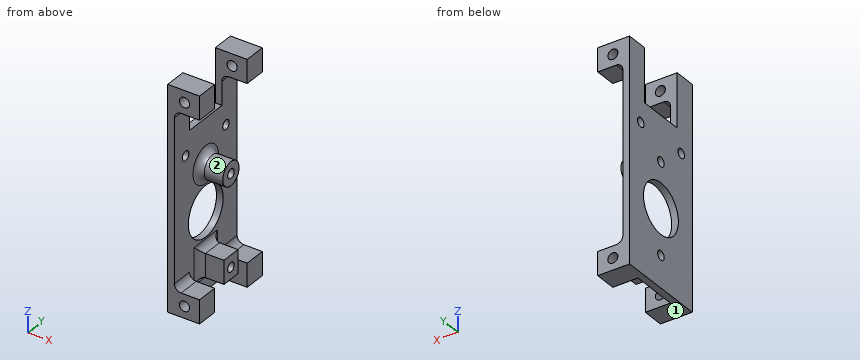
```python
from build123d import *

# Parameters (mm, degrees)
SKETCH1_W           = 66
SKETCH1_H           = 27
BOSS_EXTRUDE1_DEPTH = 2
SKETCH2_R           = 7.5
CUT_EXTRUDE1_DEPTH  = 2
BOSS_EXTRUDE2_DEPTH = 7.5
SKETCH4_R           = 1.5
CUT_EXTRUDE2_DEPTH  = 31
SKETCH5_R           = 1.4
CUT_EXTRUDE3_DEPTH  = 31
SKETCH6_W           = 7
SKETCH6_H           = 27
BOSS_EXTRUDE3_DEPTH = 7.5
SKETCH7_R           = 1.5
CUT_EXTRUDE4_DEPTH  = 33.5
SKETCH8_W           = 16
SKETCH8_H           = 14
CUT_EXTRUDE5_DEPTH  = 15.75
SKETCH9_R           = 1.4
CUT_EXTRUDE6_DEPTH  = 31.5
SKETCH10_R          = 3.5
BOSS_EXTRUDE4_DEPTH = 7.5
SKETCH11_R          = 1.4
CUT_EXTRUDE7_DEPTH  = 9.5
CUT_EXTRUDE8_DEPTH  = 7.5
FILLET1_R           = 2


with BuildPart() as part:
    # Sketch1 → Boss-Extrude1 (new body)
    with BuildSketch(Plane(origin=(0, 0, 0), x_dir=(0, 0, -1), z_dir=(1, 0, 0))):
        Rectangle(SKETCH1_W, SKETCH1_H)
    extrude(amount=BOSS_EXTRUDE1_DEPTH)

    # Sketch2 → Cut-Extrude1 (cut)
    with BuildSketch(Plane(origin=(2, 0, 0), x_dir=(0, 0, -1), z_dir=(1, 0, 0))):
        with Locations((10, 0)):
            Circle(SKETCH2_R)
    extrude(amount=-CUT_EXTRUDE1_DEPTH, mode=Mode.SUBTRACT)

    # Sketch3 → Boss-Extrude2 (add)
    with BuildSketch(Plane(origin=(2, 0, 0), x_dir=(0, 0, -1), z_dir=(1, 0, 0))):
        Polygon((33, 13.5), (26, 13.5), (26, 3), (20, 3), (20, -3), (26, -3), (26, -13.5), (33, -13.5), align=None)
    extrude(amount=BOSS_EXTRUDE2_DEPTH)

    # Sketch4 → Cut-Extrude2 (cut)
    with BuildSketch(Plane(origin=(0, 13.5, 0), x_dir=(1, 0, 0), z_dir=(0, 1, 0))):
        with Locations(Location((5, 29.5, 0), (0, 0, 270))):
            Circle(SKETCH4_R)
    extrude(amount=-CUT_EXTRUDE2_DEPTH, mode=Mode.SUBTRACT)

    # Sketch5 → Cut-Extrude3 (cut)
    with BuildSketch(Plane(origin=(9.5, 0, 0), x_dir=(0, 0, -1), z_dir=(1, 0, 0))):
        with Locations((23.54, 0)):
            Circle(SKETCH5_R)
    extrude(amount=-CUT_EXTRUDE3_DEPTH, mode=Mode.SUBTRACT)

    # Sketch6 → Boss-Extrude3 (add)
    with BuildSketch(Plane(origin=(2, 0, 0), x_dir=(0, 0, -1), z_dir=(1, 0, 0))):
        with Locations((-29.5, 0)):
            Rectangle(SKETCH6_W, SKETCH6_H)
    extrude(amount=BOSS_EXTRUDE3_DEPTH)

    # Sketch7 → Cut-Extrude4 (cut)
    with BuildSketch(Plane(origin=(0, 13.5, 0), x_dir=(1, 0, 0), z_dir=(0, 1, 0))):
        with Locations(Location((5, -29.5, 0), (0, 0, 270))):
            Circle(SKETCH7_R)
    extrude(amount=-CUT_EXTRUDE4_DEPTH, mode=Mode.SUBTRACT)

    # Sketch8 → Cut-Extrude5 (cut, symmetric)
    with BuildSketch(Plane(origin=(2, 0, 0), x_dir=(0, 0, -1), z_dir=(1, 0, 0))):
        with Locations((-25, 0)):
            Rectangle(SKETCH8_W, SKETCH8_H)
    extrude(amount=CUT_EXTRUDE5_DEPTH, both=True, mode=Mode.SUBTRACT)

    # Sketch9 → Cut-Extrude6 (cut)
    with BuildSketch(Plane(origin=(2, 0, 0), x_dir=(0, 0, -1), z_dir=(1, 0, 0))):
        with Locations((-10.5, -8.7)):
            Circle(SKETCH9_R)
    cut_extrude6 = extrude(amount=-CUT_EXTRUDE6_DEPTH, mode=Mode.SUBTRACT)

    # Mirror1: Cut-Extrude6 across plane
    add(cut_extrude6.mirror(Plane.ZX), mode=Mode.SUBTRACT)

    # Sketch10 → Boss-Extrude4 (add)
    with BuildSketch(Plane(origin=(2, 0, 0), x_dir=(0, 0, -1), z_dir=(1, 0, 0))):
        with Locations(Location((-3.54, 0, 0), (0, 0, 180))):
            Circle(SKETCH10_R)
    extrude(amount=BOSS_EXTRUDE4_DEPTH)

    # Sketch11 → Cut-Extrude7 (cut)
    with BuildSketch(Plane(origin=(9.5, 0, 0), x_dir=(0, 0, -1), z_dir=(1, 0, 0))):
        with Locations((-3.54, 0)):
            Circle(SKETCH11_R)
    extrude(amount=-CUT_EXTRUDE7_DEPTH, mode=Mode.SUBTRACT)

    # Sketch12 → Cut-Extrude8 (cut)
    with BuildSketch(Plane(origin=(9.5, 0, 0), x_dir=(0, 0, -1), z_dir=(1, 0, 0))):
        Polygon((26, -7), (33, -7), (33, -3), (33, 3), (33, 7), (26, 7), (26, 3), (27, 3), (27, -3), (26, -3), align=None)
    extrude(amount=-CUT_EXTRUDE8_DEPTH, mode=Mode.SUBTRACT)

    # Fillet1
    fillet1_edges = [part.edges().sort_by_distance(p)[0] for p in [
        (2, 0, 0.04),
        (2, -10.25, 26),
        (2, -10.25, -26),
        (2, 0, -20),
        (2, -3, -23.5),
        (2, 3, -23.5),
        (2, 10.25, -26),
        (2, 10.25, 26),
        (2, 0, -27),
    ]]
    fillet(fillet1_edges, radius=FILLET1_R)


solid = part.part
```
CAD build for the part. Positions are in the model's coordinates, mm. Face numbers are marked on the shaded views. A direction names the side the tool comes from. Round coordinates to 2 decimals unless told otherwise and drop trailing zeros. Order: outer loops, then holes, each group sorted by start corner. A loop starts at its lowest first (then second) coordinate and runs counter-clockwise, first axis right, second up.
Item 1: Saw through at B-B on z = 3.54. Write the cut outline in (x, y), then the cut area to 3 significant figures.
Item 2: Tool access for the marked faces 1 and 2: list every direction of +Z, -Z, +X, -X, +Y, -Y with a clear straight run to the whole face (end or side of a thin tool).
Item 3: Saw through at D-D on y = 0. Write the cut outline in (x, z).
Item 4: Saw through at A-A on x = 7.25. Write the cut outline in (y, z), then the cut area to 3 significant figures.
Item 5: Probe line 1 along Y through (x, z) = (1.3, 10.5); line 2 along X through (y, z) = (12.25, 29.5); line 3 along Z through (x, y) = (0.4, 8.7). List the from-to ranges inside material, lowest first.
Item 6: Pin check, flat tips, straight feed: pin 1 (6 mm diameter, centred on y = 9.5, z = 3.5, fed in from +X); pin 2 (2 mm diameter, centred on x = 0.5, y = 0.5, fed in from +Z); pin 3 (2 mm diameter, centred on y = -8.7, z = 10.5, fed in from +X); pin 4 (1.6 mm diameter, centred on x = 7.5, z = -23.5, fed in from -Y). Stop position of each tip, or through.
Item 7: Saw through at C-C on y = -8.7. Write the cut outline in (x, z), then the cut area to 3 significant figures.
Reported:
1. outline: (0, -13.5) - (2, -13.5) - (2, -5.5) arc R2 cw to (4, -3.5) - (9.5, -3.5) - (9.5, -1.4) - (0, -1.4) - close; (0, 1.4) - (9.5, 1.4) - (9.5, 3.5) - (4, 3.5) arc R2 cw to (2, 5.5) - (2, 13.5) - (0, 13.5) - close
1. area: 81.6 mm2
2. face 1: -Z, +X, -X, +Y, -Y
2. face 2: +X
3. outline: (0, -33) - (2, -33) - (2, -29) arc R2 cw to (4, -27) - (9.5, -27) - (9.5, -24.94) - (0, -24.94) - close; (0, -22.14) - (9.5, -22.14) - (9.5, -20) - (4, -20) arc R2 cw to (2, -18) - (2, -17.5) - (0, -17.5) - close; (0, -2.5) - (2, -2.5) - (2, -1.96) arc R2 cw to (4, 0.04) - (9.5, 0.04) - (9.5, 2.14) - (0, 2.14) - close; (0, 4.94) - (9.5, 4.94) - (9.5, 7.04) - (4, 7.04) arc R2 cw to (2, 9.04) - (2, 17) - (0, 17) - close
4. outline: (-13.5, -33) - (-7, -33) - (-7, -26) - (-13.5, -26) - close; (-13.5, 26) - (-7, 26) - (-7, 33) - (-13.5, 33) - close; circle Ø7 at (0, 3.54); (-3, -27) - (3, -27) - (3, -20) - (-3, -20) - close; (7, -33) - (13.5, -33) - (13.5, -26) - (7, -26) - close; (7, 26) - (13.5, 26) - (13.5, 33) - (7, 33) - close; hole circle Ø2.8 at (0, -23.54); hole circle Ø2.8 at (0, 3.54)
4. area: 250 mm2
5. line 1: y = -13.5 to -10.1, -7.3 to 7.3, 10.1 to 13.5
5. line 2: x = 0 to 3.5, 6.5 to 9.5
5. line 3: z = -33 to 9.1, 11.9 to 33
6. pin 1: stops at x = 2
6. pin 2: stops at z = 17
6. pin 3: passes through
6. pin 4: stops at y = -3
7. outline: (0, -33) - (9.5, -33) - (9.5, -26) - (4, -26) arc R2 cw to (2, -24) - (2, 9.1) - (0, 9.1) - close; (0, 11.9) - (2, 11.9) - (2, 24) arc R2 cw to (4, 26) - (9.5, 26) - (9.5, 33) - (0, 33) - close; hole circle Ø3 at (5, -29.5); hole circle Ø3 at (5, 29.5)
7. area: 219 mm2
